from build123d import *

# Parameters (mm, degrees)
SKETCH_2_R          = 13.5
CUT_EXTRUDE_1_DEPTH = 26.228951623
SKETCH_3_W          = 2.58
SKETCH_3_H          = 12
CHAMFER_1_SIZE      = 0.3


with BuildPart() as part:
    # 草图1 → 旋转1 (revolve)
    with BuildSketch(Plane.XY):
        with BuildLine():
            Line((0, 0), (-7.5, 0))
            Line((-7.5, 0), (-7.5, 10.8))
            ThreePointArc((-7.5, 10.8), (-10.020409182, 11.359397565), (-12.5, 12.078436826))
            Line((-12.5, 12.078436826), (-12.5, 15.795912741))
            ThreePointArc((-12.5, 15.795912741), (-6.346416324, 17.444760518), (0, 18))
            Line((0, 18), (0, 0))
        make_face()
    revolve(axis=Axis((0, 18, 0), (0, -1, 0)))

    # 草图2 → 切除-拉伸1 (cut, through all)
    with BuildSketch(Plane(origin=(0, 0, 0), x_dir=(1, 0, 0), z_dir=(0, 1, 0))):
        Circle(SKETCH_2_R)
        with BuildLine():
            ThreePointArc((2.301292124, 10.976757166), (0, 12.5), (-2.301292124, 10.976757166))
            ThreePointArc((-2.301292124, 10.976757166), (-5.266555861, 7.24879227), (-9.728378055, 5.580663378))
            ThreePointArc((-9.728378055, 5.580663378), (-11.888206454, 3.86271243), (-11.150654806, 1.203345637))
            ThreePointArc((-11.150654806, 1.203345637), (-8.521466386, -2.76879227), (-8.313760417, -7.527717519))
            ThreePointArc((-8.313760417, -7.527717519), (-7.347315654, -10.11271243), (-4.590191543, -10.233048662))
            ThreePointArc((-4.590191543, -10.233048662), (0, -8.96), (4.590191543, -10.233048662))
            ThreePointArc((4.590191543, -10.233048662), (7.347315654, -10.11271243), (8.313760417, -7.527717519))
            ThreePointArc((8.313760417, -7.527717519), (8.521466386, -2.76879227), (11.150654806, 1.203345637))
            ThreePointArc((11.150654806, 1.203345637), (11.888206454, 3.86271243), (9.728378055, 5.580663378))
            ThreePointArc((9.728378055, 5.580663378), (5.266555861, 7.24879227), (2.301292124, 10.976757166))
        make_face(mode=Mode.SUBTRACT)
    extrude(amount=CUT_EXTRUDE_1_DEPTH, mode=Mode.SUBTRACT)

    # 草图3 → 切除-旋转1 (revolve, cut)
    with BuildSketch(Plane.XY, mode=Mode.PRIVATE) as cut_revolve_1_sk:
        with Locations((1.29, 6)):
            Rectangle(SKETCH_3_W, SKETCH_3_H)
    revolve(cut_revolve_1_sk.sketch.rotate(Axis((0, 0, 0), (0, 1, 0)), 173.840646027), axis=Axis((0, 0, 0), (0, 1, 0)), mode=Mode.SUBTRACT)

    # 倒角1
    chamfer_1_edges = [part.edges().sort_by_distance(p)[0] for p in [
        (7.5, 0, 0),
    ]]
    chamfer(chamfer_1_edges, length=CHAMFER_1_SIZE)


solid = part.part
Build history of the part. All positions in model axes, mm. A direction names the side the tool comes from. Give positions to 0.01 mm unless a question says otherwise; leave off trailing zeros. Loops run counter-clockwise (first coordinate to the right, second up) from the corner with the lowest first, then second, coordinate; pieces in that order, holes last. Notation, with made-up numbers: (-28, 5) -> (-9, 5) arc R31 ccw to (-9, 44) -> close; hole circle Ø1 at (-9.5, 21.25). An arc over 180 degrees is marked (long way). Answer in a Markdown table with one row per item.
Item 1: Slice it at B-B on y = 13.75. Write the cut outline in (x, z), plus the area to 3 significant figures.
Findings below:
| item | result |
|---|---|
| outline | (-11.15, -1.2) arc R2.5 ccw to (-9.73, -5.58) arc R8.91 cw to (-2.3, -10.98) arc R2.5 ccw to (2.3, -10.98) arc R8.91 cw to (9.73, -5.58) arc R2.5 ccw to (11.15, -1.2) arc R8.91 cw to (8.31, 7.53) arc R2.5 ccw to (4.59, 10.23) arc R8.91 cw to (-4.59, 10.23) arc R2.5 ccw to (-8.31, 7.53) arc R8.91 cw to start |
| area | 347 mm² |
Item 2: Tool access for faces 4 (the cylindrical face through (11.9, 13.93, -3.82)), 5 (the cylindrical face through (7.493, 5.624, -0.33)): list every direction of +Z, -Z, +X, -X, +Y, -Y with a clear straight run to the whole face (end or side of a thin tool).
Findings below:
| item | result |
|---|---|
| face 4 | +X, +Y, -Y |
| face 5 | -Y |
Item 3: Flat gauge pins, fed straight in: P1, Ø3, axis at x = -8, y = 2, coming from the +Z side; P2, Ø6, axis at x = -1, z = -5.5, coming from the +Y side; P3, Ø5, axis at y = 7, z = 2.5, coming from the -X side. Where does each tip first touch, or does it go through?
Findings below:
| item | result |
|---|---|
| P1 | stops at z = 3.74 |
| P2 | stops at y = 17.91 |
| P3 | stops at x = -7.5 |
Item 4: Slice it at C-C on z = -10.5. Write the cut outline in (x, y).
Findings below:
| item | result |
|---|---|
| outline | (-2.52, 11.57) arc R39.06 ccw to (2.52, 11.57) -> (2.52, 16.37) arc R35.01 ccw to (-2.52, 16.37) -> close |
Item 5: Slice it at A-A on x = 0. Write the cut outline in (y, z), plus the area to 3 significant figures.
Findings below:
| item | result |
|---|---|
| outline | (0, -7.2) -> (0.3, -7.5) -> (10.8, -7.5) arc R40.45 ccw to (12.08, -12.5) -> (15.8, -12.5) arc R36.55 ccw to (16.88, 8.96) -> (11.1, 8.96) arc R40.45 ccw to (10.8, 7.5) -> (0.3, 7.5) -> (0, 7.2) -> (0, 2.58) -> (12, 2.58) -> (12, -2.58) -> (0, -2.58) -> close |
| area | 239 mm² |
Item 6: Probe line 1 along Z through (x, y) = (0, 5.5); line 2 along X through (y, z) = (8, 0.5). List the from-to ranges inside material, lowest first. Write a range as [from, to].
Findings below:
| item | result |
|---|---|
| line 1 | z = [-7.5, -2.58], [2.58, 7.5] |
| line 2 | x = [-7.48, -2.53], [2.53, 7.48] |
Item 7: Slice it at D-D on y = 10. Write the cut outline in (x, z).
Findings below:
| item | result |
|---|---|
| outline | circle Ø15 at (0, 0); hole circle Ø5.16 at (0, 0) |
Item 8: Mould opens along Z. For faces 1 (the flat face through (0, 12, 0)), 2 (the flat face through (0, 0, 3)), 3 (the cylindrical face through (-5.2, 14, -7.3)) say: pulls with the +Z half, pulls with the -Z half, needs draft (parallel to the pull), parting line crosses it, or undercut.
Findings below:
| item | result |
|---|---|
| face 1 | undercut |
| face 2 | needs draft |
| face 3 | pulls with the -Z half |
